from build123d import *

# Parameters (mm, degrees)
F0_W     = 1110
F0_H     = 750
F0_W_2   = 265
F0_H_2   = 175
F1_DEPTH = 170


with BuildPart() as f1:
    # F0 (on Front) → F1 (new body, symmetric)
    with BuildSketch(Plane.XZ):
        Rectangle(F0_W, F0_H)
        with Locations((-412.5, -277.5)):
            Rectangle(F0_W_2, F0_H_2, mode=Mode.SUBTRACT)
        with Locations((-137.5, -277.5)):
            Rectangle(F0_W_2, F0_H_2, mode=Mode.SUBTRACT)
        with Locations((-412.5, -92.5)):
            Rectangle(F0_W_2, F0_H_2, mode=Mode.SUBTRACT)
        with Locations((-137.5, -92.5)):
            Rectangle(F0_W_2, F0_H_2, mode=Mode.SUBTRACT)
        with Locations((137.5, -277.5)):
            Rectangle(F0_W_2, F0_H_2, mode=Mode.SUBTRACT)
        with Locations((412.5, -277.5)):
            Rectangle(F0_W_2, F0_H_2, mode=Mode.SUBTRACT)
        with Locations((137.5, -92.5)):
            Rectangle(F0_W_2, F0_H_2, mode=Mode.SUBTRACT)
        with Locations((412.5, -92.5)):
            Rectangle(F0_W_2, F0_H_2, mode=Mode.SUBTRACT)
        with Locations((-412.5, 92.5)):
            Rectangle(F0_W_2, F0_H_2, mode=Mode.SUBTRACT)
        with Locations((-137.5, 92.5)):
            Rectangle(F0_W_2, F0_H_2, mode=Mode.SUBTRACT)
        with Locations((-412.5, 277.5)):
            Rectangle(F0_W_2, F0_H_2, mode=Mode.SUBTRACT)
        with Locations((-137.5, 277.5)):
            Rectangle(F0_W_2, F0_H_2, mode=Mode.SUBTRACT)
        with Locations((137.5, 92.5)):
            Rectangle(F0_W_2, F0_H_2, mode=Mode.SUBTRACT)
        with Locations((412.5, 92.5)):
            Rectangle(F0_W_2, F0_H_2, mode=Mode.SUBTRACT)
        with Locations((137.5, 277.5)):
            Rectangle(F0_W_2, F0_H_2, mode=Mode.SUBTRACT)
        with Locations((412.5, 277.5)):
            Rectangle(F0_W_2, F0_H_2, mode=Mode.SUBTRACT)
    extrude(amount=F1_DEPTH, both=True)


solid = f1.part
Input: part model. Units: mm. Frame: model coordinates. Coordinates: 2 decimals unless noted, no trailing zeros. Order: outer loops, then holes, each group sorted by start corner. A loop starts at its lowest first (then second) coordinate and runs counter-clockwise, first axis right, second up.
1. Ray query, line 1 along Z through (x, y) = (-15, 46); line 2 along X through (y, z) = (-129, 311). Return the intervals inside material, ascending.
Checked values:
line 1: z = -375 to -365, -190 to -180, -5 to 5, 180 to 190, 365 to 375
line 2: x = -555 to -545, -280 to -270, -5 to 5, 270 to 280, 545 to 555
2. Cut plane A-A, the plane x = -29. Return loops of the section in (y, z), plus the area to 3 significant figures.
Checked values:
outline: (-170, -375) - (170, -375) - (170, -365) - (-170, -365) - close; (-170, -190) - (170, -190) - (170, -180) - (-170, -180) - close; (-170, -5) - (170, -5) - (170, 5) - (-170, 5) - close; (-170, 180) - (170, 180) - (170, 190) - (-170, 190) - close; (-170, 365) - (170, 365) - (170, 375) - (-170, 375) - close
area: 17,000 mm2
3. Draft query along X for faces 1 (the flat face through (-8, -2, -375)), 2 (the flat face through (-139, -2, 5)). Return one class per face: +X half, -X half, draft (parallel to the pull), parting line (faces both ways), or undercut.
Checked values:
face 1: draft
face 2: undercut
4. Cut plane C-C, the plane y = 103. Count the separate pieces of the cut face and the enclosed holes in it, plus the area to 3 significant figures.
Checked values:
separate pieces: 1
enclosed holes: 16
area: 90,500 mm2
5. Cut plane B-B, the plane z = 36.5. Return loops of the section in (x, y).
Checked values:
outline: (-555, -170) - (-545, -170) - (-545, 170) - (-555, 170) - close; (-280, -170) - (-270, -170) - (-270, 170) - (-280, 170) - close; (-5, -170) - (5, -170) - (5, 170) - (-5, 170) - close; (270, -170) - (280, -170) - (280, 170) - (270, 170) - close; (545, -170) - (555, -170) - (555, 170) - (545, 170) - close
